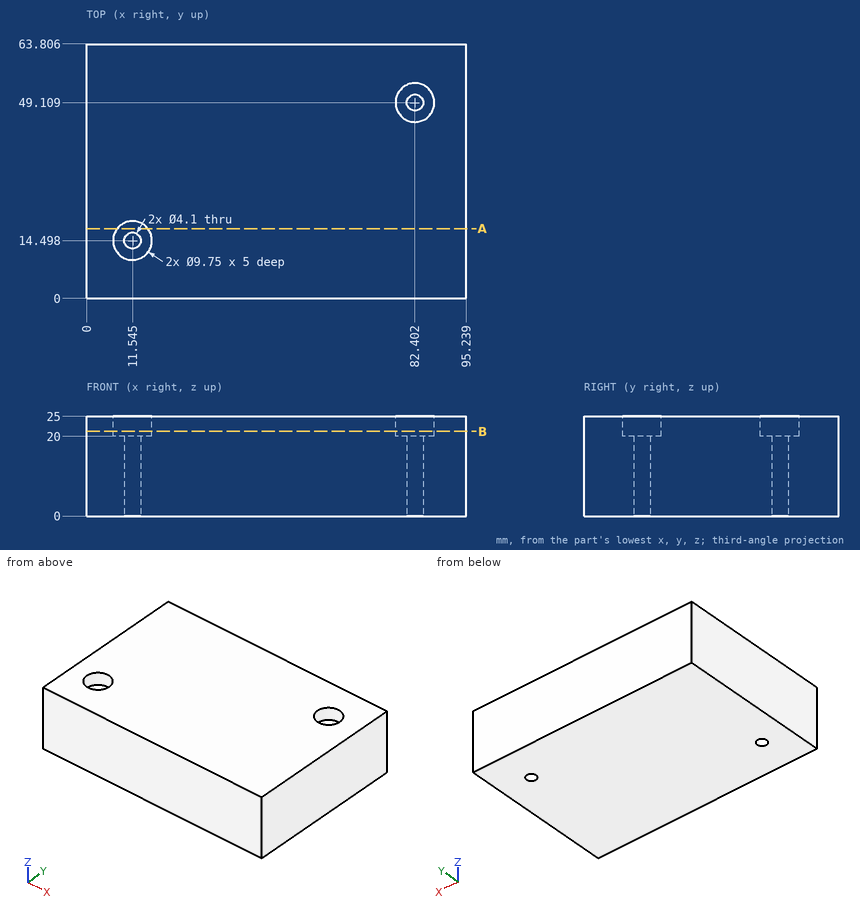
Could you check a few things on this drawing? It's one solid part, dimensions in mm from its lowest x, y, z. Give positions to 0.01 mm unless a question says otherwise; leave off trailing zeros. Order: outer loops, then holes, each group sorted by start corner. A loop starts at its lowest first (then second) coordinate and runs counter-clockwise, first axis right, second up. Notation, with made-up numbers: M 33,-20.5 L 60,-20.5 A26 cw 60,0.5 Z; hole C 31,87.5 d10. An arc over 180 degrees is marked long. Use one line per item in the form item = value. Start each with the question number.
Item 1: Will this pin go through, and if not, where does the flat tip stop? pin 1 Ø3 at (x, y) = (80, 48.5) entering from +Z.
Item 2: If I drill on line 1 along X through (y, z) = (16, 1.25), over which ranges is the centre line in solid material (lowest first)?
Item 3: If we section it at B-B (z = 21.25): State how many separate pieces and enclosed holes the cut face has, then the cut area to 3 significant figures.
Item 4: If we section it at A-A (y = 17.5): Write out the boundary of the cut face in (x, z), then the cut area to 3 significant figures.
Outcome:
q1.pin_1 = 20
q2.line_1 = 0 to 10.15, 12.94 to 95.24
q3.separate_pieces = 1
q3.enclosed_holes = 2
q3.area = 5,930 mm2
q4.outline = M 0,0 L 95.24,0 L 95.24,25 L 15.39,25 L 15.39,20 L 7.7,20 L 7.7,25 L 0,25 Z
q4.area = 2,340 mm2
